Part model, mm, in its own coordinate system. Coordinates: 2 decimals unless noted, no trailing zeros. Loops run counter-clockwise (first coordinate to the right, second up) from the corner with the lowest first, then second, coordinate; pieces in that order, holes last. Notation, with made-up numbers: (13, -11.5) - (19, -11.5) arc R6 cw to (19, -0.5) - close; hole circle Ø7 at (80.5, 74.5). An arc over 180 degrees is marked (long way). Answer as CSV lines item,"result".
Autodesk Inventor part; units mm, degrees
ref_plane "YZ Plane" through (0, 0, 0) normal (1, 0, 0) x (0, 1, 0)
ref_plane "XZ Plane" through (0, 0, 0) normal (0, 1, 0) x (-1, 0, 0)
ref_plane "XY Plane" through (0, 0, 0) normal (0, 0, 1) x (1, 0, 0)
sketch "Esboço1" plane through (0, 0, 0) normal (0, 1, 0) x (-1, 0, 0)
  line L0 (0, 0) -> (80, 0)
  line L1 (80, 0) -> (80, -80)
  line L2 (80, -80) -> (0, -80)
  line L3 (0, -80) -> (0, 0)
  circle A0 centre (40, -40) radius 6
  dimension "d0" = 80
  dimension "d1" = 80
  dimension "d2" = 12
extrude "Extrusão1" add sketch "Esboço1" along normal blind 12
fillet "Arredondamento1" radius 10 4 edges at (-80, 6, 0) (0, 6, 0) (0, 6, -80) (-80, 6, -80)
properties part number "Calorímetro_montagem"
Q1. Two-plate mould, pull along Z, no slides. Class faces 1 (the face through (-77.15, 6.08, -3.01)), 2 (the face through (-35.24, 5.92, -36.35)), 3 (the face through (-80, 6, -40)), 4 (the face through (-2.85, 6.08, -76.99)): released by +Z, released by -Z, zero draft, split by the parting line, or undercut.
Results:
face 1,"released by +Z"
face 2,"undercut"
face 3,"zero draft"
face 4,"released by -Z"
Q2. Saw through at B-B (z = -40). Give the cut face in (x, y), then the cut area to 3 significant figures.
Results:
outline,"(-80, 0) - (-46, 0) - (-46, 12) - (-80, 12) - close; (-34, 0) - (0, 0) - (0, 12) - (-34, 12) - close"
area,"816 mm^2"
Q3. Saw through at A-A (x = -40). Give the cut face in (y, z).
Results:
outline,"(0, -80) - (12, -80) - (12, -46) - (0, -46) - close; (0, -34) - (12, -34) - (12, 0) - (0, 0) - close"
Q4. Saw through at C-C (y = 5.5). Give the cut face in (x, z).
Results:
outline,"(-80, -70) arc R10 ccw to (-70, -80) - (-10, -80) arc R10 ccw to (0, -70) - (0, -10) arc R10 ccw to (-10, 0) - (-70, 0) arc R10 ccw to (-80, -10) - close; hole circle Ø12 at (-40, -40)"
Q5. Wall check: L1, parallel to Z at x = -40, y = 4.5; L2, parallel to X at y = 3, z = -37; L3, parallel to Z at x = -36, y = 1.75. Give the ranges that are in metal, low to high.
Results:
L1,"z = -80 to -46, -34 to 0"
L2,"x = -80 to -45.2, -34.8 to 0"
L3,"z = -80 to -44.47, -35.53 to 0"
